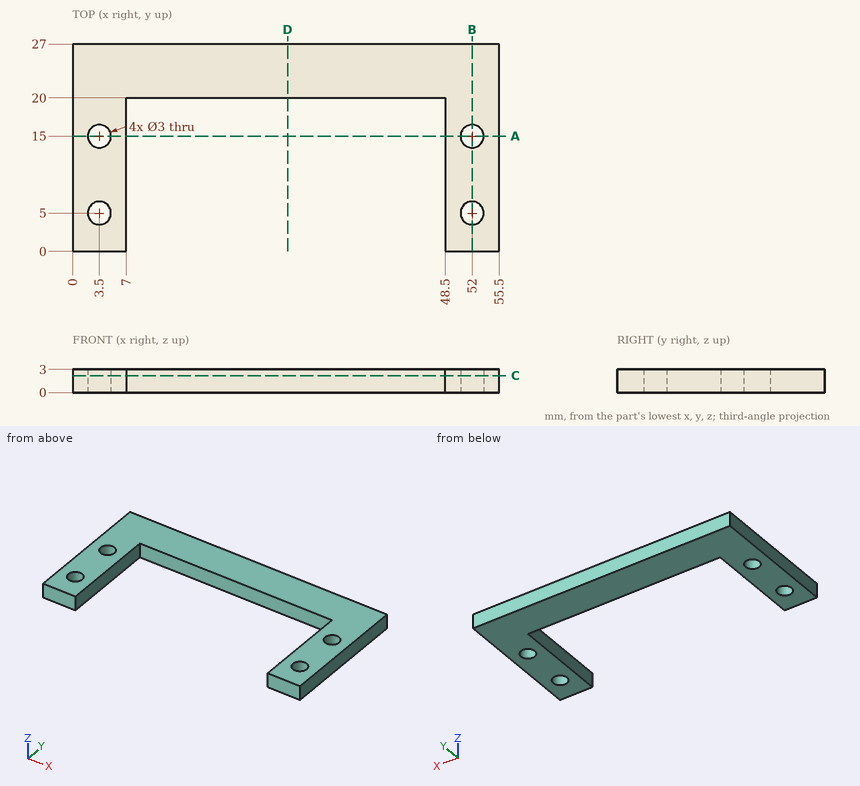
Could you check a few things on this drawing? It's one solid part, dimensions in mm from its lowest x, y, z. Round coordinates to 2 decimals unless told otherwise and drop trailing zeros. Loops run counter-clockwise (first coordinate to the right, second up) from the corner with the lowest first, then second, coordinate; pieces in that order, holes last. Notation, with made-up numbers: M 32.25,-39.75 L 63.25,-39.75 A25 cw 63.25,-14.75 Z; hole C 20.25,61.25 d10. An arc over 180 degrees is marked long. Write each question's results on one line, items separated by ' | '. Start each with the question number.
(1) I want a section at D-D (x = 28). Please give me the cut outline in (y, z).
(2) I want a section at A-A (y = 15). Please give me the cut outline in (x, z), then the cut area to 3 significant figures.
(3) Will these pins go through, and if not, where does the flat tip stop? P1, Ø5, axis at x = 3.5, y = 15, coming from the +Z side; P2, Ø0.9, axis at x = 31, z = 1, coming from the -Y side.
(4) If I drill on probe 1 along Y at (x, z) = (3.5, 2.3); probe 2 along X at (y, z) = (11.75, 2.7); probe 3 along Y at (x, z) = (52.5, 2), over which ranges is the centre line in solid material (lowest first)? Write a range as from..to.
(5) I want a section at C-C (z = 2.2). Please give me the cut outline in (x, y).
(6) I want a section at B-B (x = 52). Please give me the cut outline in (y, z).
Solved:
1) outline: M 20,0 L 27,0 L 27,3 L 20,3 Z
2) outline: M 0,0 L 2,0 L 2,3 L 0,3 Z; M 5,0 L 7,0 L 7,3 L 5,3 Z; M 48.5,0 L 50.5,0 L 50.5,3 L 48.5,3 Z; M 53.5,0 L 55.5,0 L 55.5,3 L 53.5,3 Z | area: 24.0 mm²
3) P1: stops at z = 3 | P2: stops at y = 20
4) probe 1: y = 0..3.5, 6.5..13.5, 16.5..27 | probe 2: x = 0..7, 48.5..55.5 | probe 3: y = 0..3.59, 6.41..13.59, 16.41..27
5) outline: M 0,0 L 7,0 L 7,20 L 48.5,20 L 48.5,0 L 55.5,0 L 55.5,27 L 0,27 Z; hole C 3.5,5 d3; hole C 3.5,15 d3; hole C 52,5 d3; hole C 52,15 d3
6) outline: M 0,0 L 3.5,0 L 3.5,3 L 0,3 Z; M 6.5,0 L 13.5,0 L 13.5,3 L 6.5,3 Z; M 16.5,0 L 27,0 L 27,3 L 16.5,3 Z
